from build123d import *

# Parameters (mm, degrees)
SKETCH_2_W                   = 295
SKETCH_2_H                   = 15
EXTRUDE_1_DEPTH              = 27
PATTERN_LINEAR_1_COUNT       = 12
PATTERN_LINEAR_1_PITCH       = 25
CUT_EXTRUDE_1_REACH          = 298.37
SKETCH_6_W                   = 12
SKETCH_6_H                   = 2
HOLE_WIZARD_M4_1_D           = 4.5
HOLE_WIZARD_M4_1_CBORE_D     = 8
HOLE_WIZARD_M4_1_CBORE_DEPTH = 4.5
PATTERN_LINEAR_2_COUNT       = 11
PATTERN_LINEAR_2_PITCH       = 25


with BuildPart() as part:
    # 草图2 → 拉伸1 (new body)
    with BuildSketch(Plane(origin=(0, 0, 0), x_dir=(1, 0, 0), z_dir=(0, 1, 0))):
        with Locations((147.5, -1.5)):
            Rectangle(SKETCH_2_W, SKETCH_2_H)
    extrude(amount=EXTRUDE_1_DEPTH)

    # 草图4 → M3 螺纹孔1 (revolve, cut)
    with BuildSketch(Plane(origin=(10, 27, 0), x_dir=(0, 0, 1), z_dir=(1, 0, 0))):
        Polygon((0, 0), (0, 8.251075774), (1.25, 7.5), (1.25, 0), align=None)
    hole_wizard_m3_1 = revolve(axis=Axis((10, 33.35, 0), (0, -1, 0)), mode=Mode.SUBTRACT)

    # 阵列(线性)1: M3 螺纹孔1 ×12
    with Locations(*[(i * PATTERN_LINEAR_1_PITCH, 0, 0) for i in range(1, PATTERN_LINEAR_1_COUNT)]):
        add(hole_wizard_m3_1, mode=Mode.SUBTRACT)

    # 草图6 → 切除-拉伸1 (cut, up to next)
    with BuildSketch(Plane(origin=(295, 0, 0), x_dir=(0, 0, -1), z_dir=(1, 0, 0)), mode=Mode.PRIVATE) as cut_extrude_1_sk1:
        with Locations((0, 26)):
            Rectangle(SKETCH_6_W, SKETCH_6_H)
    cut_extrude_1_tool1 = extrude(cut_extrude_1_sk1.sketch, amount=-CUT_EXTRUDE_1_REACH, mode=Mode.PRIVATE) & part.part
    add(cut_extrude_1_tool1.solids().sort_by_distance((295, 26, 0))[0], mode=Mode.SUBTRACT)

    # M4 六角凹头螺钉的柱形沉头孔1 (through all)
    with Locations(Plane(origin=(0, 25, 0), x_dir=(-1, 0, 0), z_dir=(0, 1, 0))):
        with Locations((-22.5, 0)):
            hole_wizard_m4_1 = CounterBoreHole(HOLE_WIZARD_M4_1_D / 2, HOLE_WIZARD_M4_1_CBORE_D / 2, HOLE_WIZARD_M4_1_CBORE_DEPTH)

    # 阵列(线性)2: M4 六角凹头螺钉的柱形沉头孔1 ×11
    with Locations(*[(i * PATTERN_LINEAR_2_PITCH, 0, 0) for i in range(1, PATTERN_LINEAR_2_COUNT)]):
        add(hole_wizard_m4_1, mode=Mode.SUBTRACT)


solid = part.part
The listing builds one solid part. Answer for the finished solid, in the listing's coordinates (mm). A direction names the side the tool comes from. Give positions to 0.01 mm unless a question says otherwise; leave off trailing zeros. Loops run counter-clockwise (first coordinate to the right, second up) from the corner with the lowest first, then second, coordinate; pieces in that order, holes last. Notation, with made-up numbers: (-23, 19.5) - (9, 19.5) arc R33 cw to (9, 50.5) - close; hole circle Ø7 at (60, 78.25). An arc over 180 degrees is marked (long way). Write each question's results on one line, items separated by ' | '.
1. Find section B-B, the plane x = 204. Write down the section's boundary in (y, z).
Resolved:
outline: (0, -6) - (25, -6) - (25, 6) - (27, 6) - (27, 9) - (0, 9) - close
2. Which of the six approach directions +Z, -Z, +X, -X, +Y, -Y give full straight-line access (tool end or side, diameter ignored) to faces 4 (the face through (145, 12, -6)), 5 (the face through (46, 20.5, -2))?
Resolved:
face 4: -Z, +X, -X, +Y, -Y | face 5: +Y
3. Flat-ended cylindrical pins translate along their axes: P1, Ø7, axis at x = 247.5, z = 0, coming from the +Y side; P2, Ø9, axis at x = 223.5, z = -0.5, coming from the +Y side; P3, Ø2, axis at x = 10, z = 0, coming from the +Y side. Find the tip coordinate at first contact, or state that the pin passes through.
Resolved:
P1: stops at y = 20.5 | P2: stops at y = 25 | P3: stops at y = 19.35
4. Consider probe 1 along Z at (x, y) = (47.5, 23.25); probe 2 along Z at (x, y) = (72, 9.75); probe 3 along Y at (x, z) = (202.5, 4.25). Determine where each line is inside the solid, lowest interval first. Write a range as from..to.
Resolved:
probe 1: z = -6..-4, 4..9 | probe 2: z = -6..-2.19, 2.19..9 | probe 3: y = 0..25
5. Find section A-A, the plane y = 6.5. Count the separate pieces of the cut face and the enclosed holes in it, then the cut area to 3 significant figures.
Resolved:
separate pieces: 1 | enclosed holes: 11 | area: 4,250 mm^2
6. For a pull along Z with two mould halves and no side action, classify faces 1 (the face through (0, 13, 2)), 2 (the face through (174.58, 10.11, -0.86)), 3 (the face through (145, 13, 9)) as +Z half, -Z half, draft (parallel to the pull), parting line (faces both ways), or undercut.
Resolved:
face 1: draft | face 2: undercut | face 3: +Z half
